Autodesk Inventor part; units mm, degrees
ref_plane "YZ Plane" through (0, 0, 0) normal (1, 0, 0) x (0, 1, 0)
ref_plane "XZ Plane" through (0, 0, 0) normal (0, 1, 0) x (-1, 0, 0)
ref_plane "XY Plane" through (0, 0, 0) normal (0, 0, 1) x (1, 0, 0)
sketch "Sketch1" plane through (0, 0, 0) normal (0, 1, 0) x (-1, 0, 0)
  circle A0 centre (0, 0) radius 9.525
  dimension "d0" = 19.05
extrude "Extrusion1" add sketch "Sketch1" along normal blind 1.016
sketch "Sketch2" plane through (0, 1.016, 0) normal (0, 1, 0) x (1, 0, 0)
  circle A0 centre (0, 0) radius 9.525
  circle A1 centre (0, 0) radius 12.7
  dimension "d3" = 25.4
extrude "Extrusion2" add sketch "Sketch2" along normal blind 11.684 contours A0 | A1
hole "Hole1" at (0, 12.7, 0) direction (0, -1, 0) diameter 6.35 end through all
properties part number "Wing-Nut-Spacing-Test"
Geometry: final body of the model. Coordinates: model frame, mm. A direction names the side the tool comes from. Round coordinates to 2 decimals unless told otherwise and drop trailing zeros. Write each loop counter-clockwise with the first axis right and the second up, starting at its lowest first coordinate (ties: lowest second). Pieces come first, ordered by that corner, then holes. Notation, with made-up numbers: (-35, -38.75) -> (14, -38.75) arc R23 ccw to (14, -16.75) -> close; hole circle Ø9 at (76.5, 49). An arc over 180 degrees is marked (long way). Return JSON: item names as keys, results as strings.
Q1. First-contact query: pin 1 Ø3 at (x, y) = (-6, 10.5) entering from -Z; pin 2 Ø4 at (y, z) = (5.5, -5) entering from +X. Flat tips, straight axial feed; report the tip coordinate or a pass-through.
From the geometry:
{"pin 1": "z = -11.88", "pin 2": "x = 12.34"}
Q2. Ray query, line 1 (X direction, y = 6.25, z = 0) (3 decimals); line 2 (Z direction, x = 2, y = 7). Return the intervals inside material, ascending.
From the geometry:
{"line 1": "-12.7 to -3.175, 3.175 to 12.7", "line 2": "-12.54 to -2.47, 2.47 to 12.54"}
Q3. Section A-A on z = 0. Return the cut outline in (x, y) (3 decimals), and give its area (3 significant figures).
From the geometry:
{"outline": "(-12.7, 1.016) -> (-9.525, 1.016) -> (-9.525, 0) -> (-3.175, 0) -> (-3.175, 12.7) -> (-12.7, 12.7) -> close; (3.175, 0) -> (9.525, 0) -> (9.525, 1.016) -> (12.7, 1.016) -> (12.7, 12.7) -> (3.175, 12.7) -> close", "area": "235 mm2"}
Q4. Mould query, pull axis X, two halves, no side actions, for faces 3 (the cylindrical face through (7.559, 0.501, 5.796)), 4 (the cylindrical face through (3.1, 6.26, -0.69)), 5 (the flat face through (-4, 0, 0)). Classes: +X half, -X half, draft (parallel to the pull), parting line (faces both ways), or undercut.
From the geometry:
{"face 3": "parting line", "face 4": "undercut", "face 5": "draft"}
Q5. Section C-C on y = 11.75. Return the cut outline in (x, z) (3 decimals).
From the geometry:
{"outline": "circle Ø25.4 at (0, 0); hole circle Ø6.35 at (0, 0)"}
Q6. Set-up query: faces 1 (the flat face through (5, 1.016, -9)), 2 (the cylindrical face through (-2.75, 6.78, -12.4)). Return all of +Z, -Z, +X, -X, +Y, -Y with unobstructed straight access to the full face (end or side cutting, diameter ignored); none if empty.
From the geometry:
{"face 1": "-Y", "face 2": "+Y, -Y"}
Q7. Section D-D on z = 8. Return the cut outline in (x, y).
From the geometry:
{"outline": "(-9.86, 1.02) -> (-5.17, 1.02) -> (-5.17, 0) -> (5.17, 0) -> (5.17, 1.02) -> (9.86, 1.02) -> (9.86, 12.7) -> (-9.86, 12.7) -> close"}
Q8. Section B-B on x = 0. Return the cut outline in (y, z) (3 decimals).
From the geometry:
{"outline": "(0, -9.525) -> (1.016, -9.525) -> (1.016, -12.7) -> (12.7, -12.7) -> (12.7, -3.175) -> (0, -3.175) -> close; (0, 3.175) -> (12.7, 3.175) -> (12.7, 12.7) -> (1.016, 12.7) -> (1.016, 9.525) -> (0, 9.525) -> close"}
